```python
from build123d import *

# Parameters (mm, degrees)
Y_KSEKLIK_EKSTR_ZYON1_DEPTH = 50
RADYUS1_R                   = 5
KES_EKSTR_ZYON1_DEPTH       = 10
KES_EKSTR_ZYON2_REACH       = 79.382
KES_EKSTR_ZYON2_END_RADIUS  = 18
IZIM4_R                     = 2.5
IZIM5_R                     = 5
KES_EKSTR_ZYON3_DEPTH       = 26
RADYUS2_R                   = 12
RADYUS3_R                   = 2


with BuildPart() as part:
    # Çizim2 → Yükseklik-Ekstrüzyon1 (new body)
    with BuildSketch(Plane(origin=(0, 0, 0), x_dir=(0, 0, -1), z_dir=(1, 0, 0))):
        with BuildLine():
            Line((-18, 0), (-48, 0))
            Line((-48, 0), (-48, 40))
            Line((-48, 40), (-38, 40))
            Line((-38, 40), (-38, 10))
            Line((-38, 10), (-26.153393661, 10))
            ThreePointArc((-26.153393661, 10), (0, 28), (26.153393661, 10))
            Line((26.153393661, 10), (52, 10))
            Line((52, 10), (52, 0))
            Line((52, 0), (28, 0))
            Line((28, 0), (18, 0))
            ThreePointArc((18, 0), (0, 18), (-18, 0))
        make_face()
    extrude(amount=-Y_KSEKLIK_EKSTR_ZYON1_DEPTH)

    # Radyus1
    radyus1_edges = [part.edges().sort_by_distance(p)[0] for p in [
        (0, 40, 43),
        (-50, 40, 43),
    ]]
    fillet(radyus1_edges, radius=RADYUS1_R)

    # Çizim3 → Kes-Ekstrüzyon1 (cut)
    with BuildSketch(Plane.XY.offset(48)):
        with BuildLine():
            Line((-31, 40), (-31, 25))
            ThreePointArc((-31, 25), (-25, 19), (-19, 25))
            Line((-19, 25), (-19, 40))
            Line((-19, 40), (-31, 40))
        make_face()
    extrude(amount=-KES_EKSTR_ZYON1_DEPTH, mode=Mode.SUBTRACT)

    # Kes-Ekstrüzyon2: up to this cylinder (the profile starts outside it)
    kes_ekstr_zyon2_end = Plane(origin=(-25, 0, 0), z_dir=(1, 0, 0)) * Cylinder(KES_EKSTR_ZYON2_END_RADIUS, 195.764, mode=Mode.PRIVATE)
    # Çizim4 → Kes-Ekstrüzyon2 (cut, up to the surface)
    with BuildSketch(Plane(origin=(0, 28, 0), x_dir=(1, 0, 0), z_dir=(0, 1, 0)), mode=Mode.PRIVATE) as kes_ekstr_zyon2_sk1:
        with Locations(Location((-25, 0, 0), (0, 0, 270))):
            Circle(IZIM4_R)
    kes_ekstr_zyon2_tool1 = extrude(kes_ekstr_zyon2_sk1.sketch, amount=-KES_EKSTR_ZYON2_REACH, mode=Mode.PRIVATE) - kes_ekstr_zyon2_end
    add(kes_ekstr_zyon2_tool1.solids().sort_by_distance((-25, 28, 0))[0], mode=Mode.SUBTRACT)

    # Çizim5 → Kes-Ekstrüzyon3 (cut)
    with BuildSketch(Plane(origin=(0, 10, 0), x_dir=(1, 0, 0), z_dir=(0, 1, 0))):
        with Locations(Location((-38.189299203, 39, 0), (0, 0, 270))):
            Circle(IZIM5_R)
        with Locations(Location((-12.189299203, 39, 0), (0, 0, 270))):
            Circle(IZIM5_R)
    extrude(amount=-KES_EKSTR_ZYON3_DEPTH, mode=Mode.SUBTRACT)

    # Radyus2
    radyus2_edges = [part.edges().sort_by_distance(p)[0] for p in [
        (0, 5, -52),
        (-50, 5, -52),
    ]]
    fillet(radyus2_edges, radius=RADYUS2_R)

    # Radyus3
    radyus3_edges = [part.edges().sort_by_distance(p)[0] for p in [
        (-25, 10, 26.153393661),
        (-25, 10, -26.153393661),
    ]]
    fillet(radyus3_edges, radius=RADYUS3_R)


solid = part.part
```
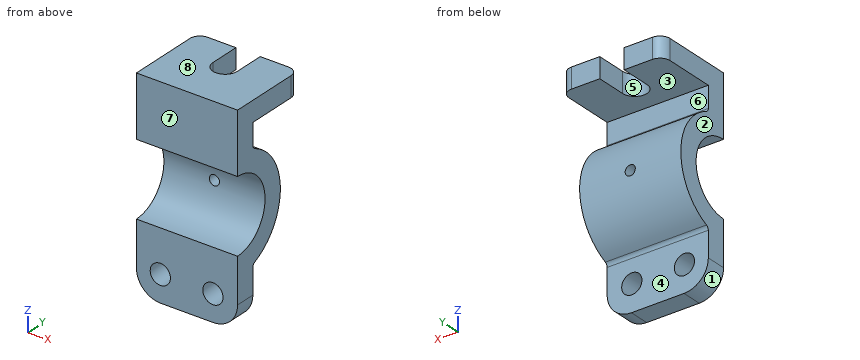
Could you check a few things on this model? Use its own coordinates, in mm. Face numbers are marked on the shaded views. A direction names the side the tool comes from. Give positions to 0.01 mm unless a question says otherwise; leave off trailing zeros. Write each loop counter-clockwise with the first axis right and the second up, starting at its lowest first coordinate (ties: lowest second). Pieces come first, ordered by that corner, then holes. Notation, with made-up numbers: (30.5, 26.5) -> (56.5, 26.5) arc R12 cw to (56.5, 40.5) -> close; hole circle Ø2 at (84.5, 58.25). An arc over 180 degrees is marked (long way). Write each question's results on one line, items separated by ' | '.
1. On a 3-axis mill with a long thin cutter (end or side, diameter ignored), from which of +Z, -Z, +X, -X, +Y, -Y can I reach the whole of each face in a straight line? I mean the marked faces 4, 5, 6, 7 and 8. Say none if no direction works.
Check sheet entries:
face 4: -Z, +X, -X, +Y | face 5: +Z, +Y | face 6: +X, -X, +Y | face 7: +Z, -Z, +X, -X, -Y | face 8: +Z, +X, -X, +Y, -Y
2. I want a section at C-C, the plane z = -39. Write out the boundary of the cut face in (x, y), then the cut area to 3 significant figures.
Check sheet entries:
outline: (-50, 0) -> (-43.19, 0) -> (-43.19, 10) -> (-50, 10) -> close; (-33.19, 0) -> (-17.19, 0) -> (-17.19, 10) -> (-33.19, 10) -> close; (-7.19, 0) -> (0, 0) -> (0, 10) -> (-7.19, 10) -> close | area: 300 mm²
3. I want a section at A-A, the plane y = 7. Write out the boundary of the cut face in (x, z).
Check sheet entries:
outline: (-50, -40) arc R12 ccw to (-38, -52) -> (-12, -52) arc R12 ccw to (0, -40) -> (0, -16.58) -> (-50, -16.58) -> close; (-50, 16.58) -> (0, 16.58) -> (0, 48) -> (-50, 48) -> close; hole circle Ø10 at (-38.19, -39); hole circle Ø10 at (-12.19, -39)
4. If we mould it in two halves opening along Z, with no side actions, what happens to the marked faces 1, 2 and 3? For each: released by +Z, released by -Z, zero draft, split by the parting line, or undercut.
Check sheet entries:
face 1: released by -Z | face 2: zero draft | face 3: undercut
5. Will these pins go through, and if not, where does the flat tip stop? pin 1 Ø7.5 at (x, z) = (-34, -37) entering from +Y; pin 2 Ø8 at (y, z) = (31, 11.5) entering from +X; pin 3 Ø10 at (x, y) = (-29, 20) entering from -Z; pin 4 Ø2 at (x, z) = (-33, 27.5) entering from +Y.
Check sheet entries:
pin 1: stops at y = 10 | pin 2: passes through | pin 3: stops at z = -23.64 | pin 4: stops at y = 10.27
6. I need wall thicknesses on L1, parallel to X at y = 2, z = -39; L2, parallel to X at y = 24.25, z = 0; L3, parallel to Z at x = -34, y = 11. Which ranges of each line are inside material? Lowest first, please.
Check sheet entries:
L1: x = -50 to -43.19, -33.19 to -17.19, -7.19 to 0 | L2: x = -50 to -27.5, -22.5 to 0 | L3: z = -25.76 to -14.25, 14.25 to 25.76, 38 to 48
7. I want a section at B-B, the plane z = 0. Write out the boundary of the cut face in (x, y), then the cut area to 3 significant figures.
Check sheet entries:
outline: (-50, 18) -> (-27.5, 18) -> (-27.5, 28) -> (-50, 28) -> close; (-22.5, 18) -> (0, 18) -> (0, 28) -> (-22.5, 28) -> close | area: 450 mm²
8. I want a section at D-D, the plane x = -35. Write out the boundary of the cut face in (y, z).
Check sheet entries:
outline: (0, -52) -> (10, -52) -> (10, -42.85) -> (0, -42.85) -> close; (0, -35.15) -> (10, -35.15) -> (10, -27.5) arc R2 cw to (11.2, -25.66) arc R28 ccw to (11.2, 25.66) arc R2 cw to (10, 27.5) -> (10, 38) -> (40, 38) -> (40, 48) -> (0, 48) -> (0, 18) arc R18 cw to (0, -18) -> close
